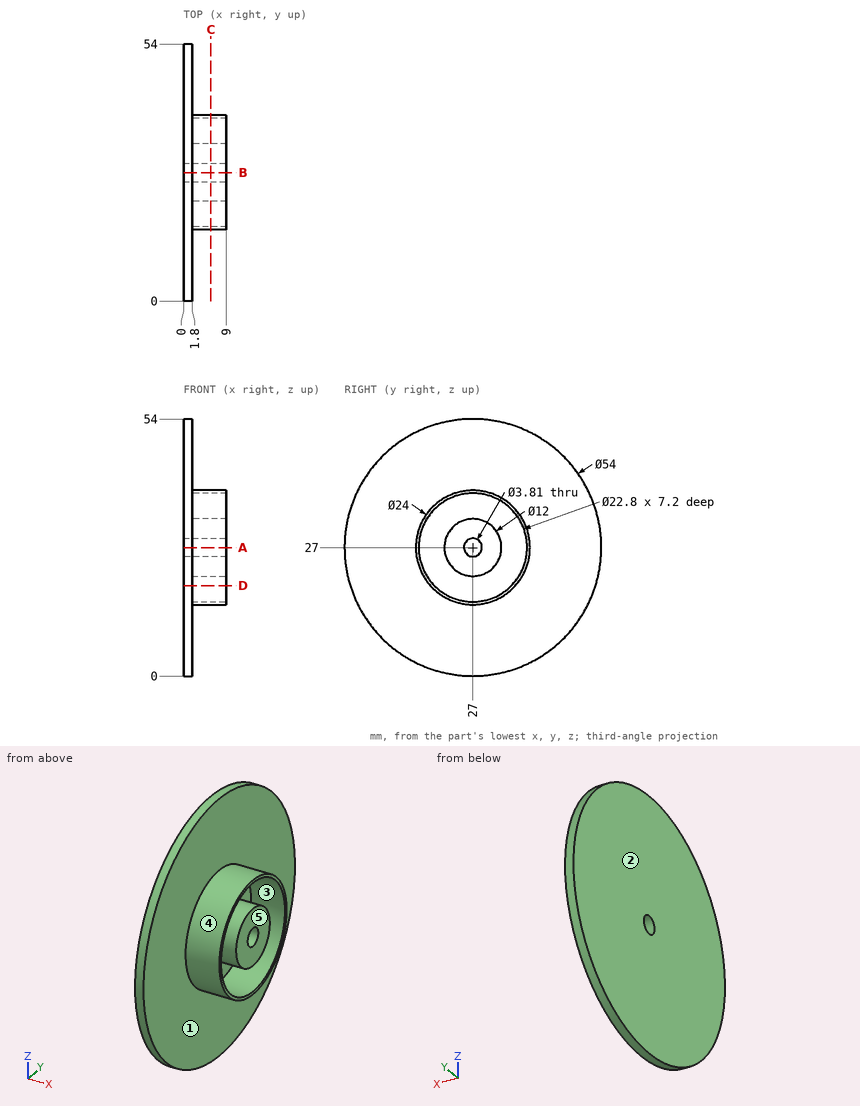
Geometry check sheet. Reference: drawing and pictorial views, mm from the part's lowest x, y, z. A direction names the side the tool comes from. Give positions to 0.01 mm unless a question says otherwise; leave off trailing zeros. Order: outer loops, then holes, each group sorted by start corner. A loop starts at its lowest first (then second) coordinate and runs counter-clockwise, first axis right, second up. Notation, with made-up numbers: M 63.5,-21.5 L 84.5,-21.5 A21 ccw 84.5,14.5 Z; hole C 39,75.25 d4. An arc over 180 degrees is marked long. Answer in a Markdown table with one row per item. Add a question column.
Item 1: Scan lines: probe 1 along Y at (x, z) = (7.75, 27) (3 decimals); probe 2 along Z at (x, y) = (3, 26). Record each from-to range of solid material in increasing order. Write a range as from..to.
Item 2: Tool access check on the marked faces 1 and 2. Record the directions out of +Z, -Z, +X, -X, +Y, -Y that give a thin tool (end or side, any length) a straight path to the whole face; none if there is none.
Item 3: Mould release check, pull along Y, two halves, no side actions. Record for the marked faces 3, 4 and 5: released by +Y, released by -Y, zero draft, split by the parting line, or undercut.
Item 4: Section check D-D, the plane z = 19. Enter the section's corners in (x, y), and give its area (3 significant figures).
Item 5: Section check C-C, the plane x = 5.75. Enter the section's corners in (y, z) (3 decimals), and give its area (3 significant figures).
Item 6: Section check A-A, the plane z = 27. Enter the section's corners in (x, y) (3 decimals), and give its area (3 significant figures).
Item 7: Gauge pin test, flat ends, axial feed: pin 1 (5 mm diameter, centred on x = 2, y = 38, fed in from +Z); pin 2 (3 mm diameter, centred on y = 35, z = 6, fed in from +X). Record the tip position at first contact, or that the pin passes through.
Filled sheet:
| question | item | result |
|---|---|---|
| 1 | probe 1 | y = 15..15.6, 21..25.095, 28.905..33, 38.4..39 |
| 1 | probe 2 | z = 15.04..15.64, 21.08..25.38, 28.62..32.92, 38.36..38.96 |
| 2 | face 1 | +X |
| 2 | face 2 | +Z, -Z, -X, +Y, -Y |
| 3 | face 3 | undercut |
| 3 | face 4 | split by the parting line |
| 3 | face 5 | zero draft |
| 4 | outline | M 0,1.21 L 1.8,1.21 L 1.8,18.06 L 9,18.06 L 9,18.88 L 1.8,18.88 L 1.8,35.12 L 9,35.12 L 9,35.94 L 1.8,35.94 L 1.8,52.79 L 0,52.79 Z |
| 4 | area | 105 mm^2 |
| 5 | outline | C 27,27 d24; C 27,27 d12; hole C 27,27 d22.8; hole C 27,27 d3.81 |
| 5 | area | 146 mm^2 |
| 6 | outline | M 0,0 L 1.8,0 L 1.8,15 L 9,15 L 9,15.6 L 1.8,15.6 L 1.8,21 L 9,21 L 9,25.095 L 0,25.095 Z; M 0,28.905 L 9,28.905 L 9,33 L 1.8,33 L 1.8,38.4 L 9,38.4 L 9,39 L 1.8,39 L 1.8,54 L 0,54 Z |
| 6 | area | 158 mm^2 |
| 7 | pin 1 | stops at z = 52.62 |
| 7 | pin 2 | stops at x = 1.8 |
